Here's the drawing with two shaded views (mm, measured from the low corner). I have some questions. A direction names the side the tool comes from. Coordinates: 2 decimals unless noted, no trailing zeros. Order: outer loops, then holes, each group sorted by start corner. A loop starts at its lowest first (then second) coordinate and runs counter-clockwise, first axis right, second up. Notation, with made-up numbers: (51, -7) -> (87, -7) arc R15 ccw to (87, 14) -> close; hole circle Ø11 at (-34, 75). An arc over 180 degrees is marked (long way). Answer as a JSON object with one key per item and string values. Group by question number.
(1) I want a section at B-B, the plane z = 0.5. List the corners of the cut face in (x, y) for me.
(2) Which directions (+Z, -Z, +X, -X, +Y, -Y) give clear straight access to the entire face, cutting with the end or side of a thin tool? Please do the marked faces 5 and 6.
(3) I want a section at C-C, the plane x = 4. List the corners of the cut face in (y, z) for me.
(4) I want a section at A-A, the plane x = 1.25. List the corners of the cut face in (y, z) for me, plus the area to 3 significant figures.
(5) If we mould it in two halves opening along Y, with no side actions, what happens to the marked faces 1, 2, 3 and 4? For each: pulls with the +Y half, pulls with the -Y half, needs draft (parallel to the pull), parting line crosses it, or undercut.
(6) I need wall thicknesses on line 1 (Y direction, x = 6.5, z = 3); line 2 (Z direction, x = 6.5, y = 8.5); line 3 (X direction, y = 8.5, z = 3). Which ranges of each line are inside material? Lowest first, please.
(7) I want a section at D-D, the plane z = 4. List the corners of the cut face in (x, y) for me, plus the area to 3 significant figures.
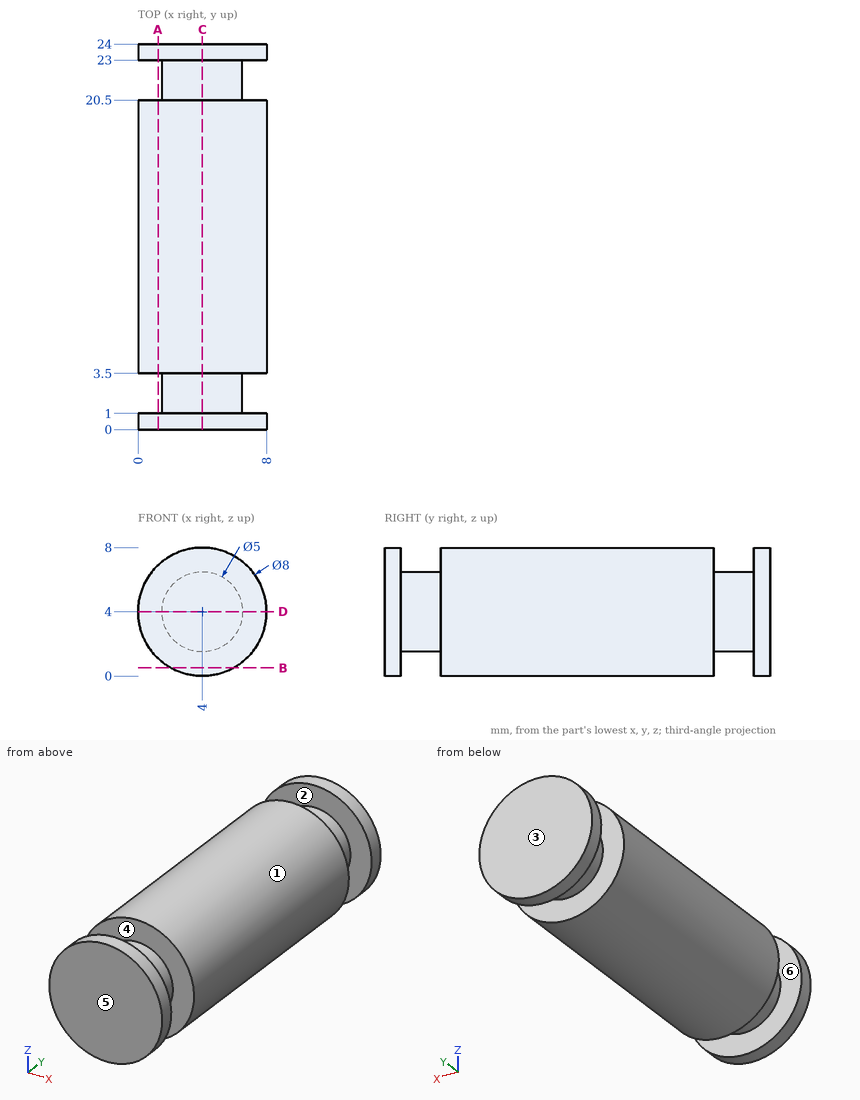
Computed values:
{
 "1": {"outline": "(2.06, 0) -> (5.94, 0) -> (5.94, 1) -> (2.06, 1) -> close; (2.06, 3.5) -> (5.94, 3.5) -> (5.94, 20.5) -> (2.06, 20.5) -> close; (2.06, 23) -> (5.94, 23) -> (5.94, 24) -> (2.06, 24) -> close"},
 "2": {"face 5": "+Z, -Z, +X, -X, -Y", "face 6": "none"},
 "3": {"outline": "(0, 0) -> (1, 0) -> (1, 1.5) -> (3.5, 1.5) -> (3.5, 0) -> (20.5, 0) -> (20.5, 1.5) -> (23, 1.5) -> (23, 0) -> (24, 0) -> (24, 8) -> (23, 8) -> (23, 6.5) -> (20.5, 6.5) -> (20.5, 8) -> (3.5, 8) -> (3.5, 6.5) -> (1, 6.5) -> (1, 8) -> (0, 8) -> close"},
 "4": {"outline": "(0, 1.1) -> (1, 1.1) -> (1, 6.9) -> (0, 6.9) -> close; (3.5, 1.1) -> (20.5, 1.1) -> (20.5, 6.9) -> (3.5, 6.9) -> close; (23, 1.1) -> (24, 1.1) -> (24, 6.9) -> (23, 6.9) -> close", "area": "110 mm2"},
 "5": {"face 1": "needs draft", "face 2": "undercut", "face 3": "pulls with the +Y half", "face 4": "undercut"},
 "6": {"line 1": "y = 0 to 1, 3.5 to 20.5, 23 to 24", "line 2": "z = 0.88 to 7.12", "line 3": "x = 0.13 to 7.87"},
 "7": {"outline": "(0, 0) -> (8, 0) -> (8, 1) -> (6.5, 1) -> (6.5, 3.5) -> (8, 3.5) -> (8, 20.5) -> (6.5, 20.5) -> (6.5, 23) -> (8, 23) -> (8, 24) -> (0, 24) -> (0, 23) -> (1.5, 23) -> (1.5, 20.5) -> (0, 20.5) -> (0, 3.5) -> (1.5, 3.5) -> (1.5, 1) -> (0, 1) -> close", "area": "177 mm2"}
}
